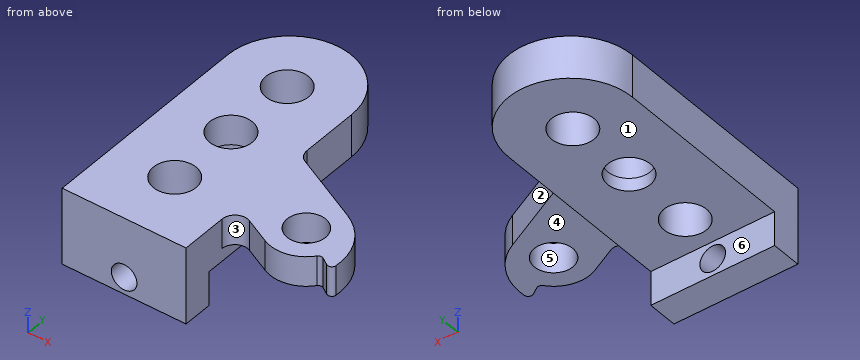
```python
from build123d import *

# Parameters (mm, degrees)
ESQUISSE1_R             = 5
ESQUISSE1_R_2           = 4.5
BOSS_EXTRU_1_DEPTH      = 7
ESQUISSE4_R             = 5
BOSS_EXTRU_3_DEPTH      = 3
ESQUISSE5_W             = 29
ESQUISSE5_H             = 7
BOSS_EXTRU_4_DEPTH      = 8
ESQUISSE6_R             = 3
ENL_V_MAT_EXTRU_1_DEPTH = 65.5
ESQUISSE8_R             = 5
ENL_V_MAT_EXTRU_2_DEPTH = 19


with BuildPart() as part:
    # Esquisse1 → Boss.-Extru.1 (new body)
    with BuildSketch(Plane.XY):
        with BuildLine():
            Line((-14.5, -25), (14.5, -25))
            Line((14.5, -25), (14.5, -14.109086144))
            ThreePointArc((14.5, -14.109086144), (15.91383086, -11.562702933), (18.822711639, -11.416423165))
            Line((18.822711639, -11.416423165), (24.752317023, -14.329211775))
            ThreePointArc((24.752317023, -14.329211775), (30.322333643, -15.002355093), (35.098387692, -12.05829076))
            ThreePointArc((35.098387692, -12.05829076), (35.719225888, -11.700832999), (36.419839787, -11.850353167))
            Line((36.419839787, -11.850353167), (38.096489271, -12.940695548))
            ThreePointArc((38.096489271, -12.940695548), (39.079315926, -13.001513562), (39.637771245, -12.190480443))
            ThreePointArc((39.637771245, -12.190480443), (37.976265411, -4.485178535), (32.247682977, 0.929211775))
            Line((32.247682977, 0.929211775), (16.177288361, 8.823440709))
            ThreePointArc((16.177288361, 8.823440709), (14.953616789, 9.929934548), (14.5, 11.516103688))
            Line((14.5, 11.516103688), (14.5, 25))
            ThreePointArc((14.5, 25), (0, 39.5), (-14.5, 25))
            Line((-14.5, 25), (-14.5, -25))
        make_face()
        with Locations((0, 7.3)):
            Circle(ESQUISSE1_R, mode=Mode.SUBTRACT)
        with Locations((28.5, -6.7)):
            Circle(ESQUISSE1_R_2, mode=Mode.SUBTRACT)
    extrude(amount=BOSS_EXTRU_1_DEPTH)

    # Esquisse4 → Boss.-Extru.3 (add)
    with BuildSketch(Plane(origin=(0, 0, 0), x_dir=(-1, 0, 0), z_dir=(0, 0, -1))):
        with BuildLine():
            Line((14.5, 25), (14.5, -25))
            Line((14.5, -25), (-14.5, -25))
            Line((-14.5, -25), (-14.5, 25))
            ThreePointArc((-14.5, 25), (0, 39.5), (14.5, 25))
        make_face()
        with Locations((0, 7.3)):
            Circle(ESQUISSE4_R, mode=Mode.SUBTRACT)
    extrude(amount=BOSS_EXTRU_3_DEPTH)

    # Esquisse5 → Boss.-Extru.4 (add)
    with BuildSketch(Plane(origin=(0, 0, -3), x_dir=(-1, 0, 0), z_dir=(0, 0, -1))):
        with Locations((0, -21.5)):
            Rectangle(ESQUISSE5_W, ESQUISSE5_H)
    extrude(amount=BOSS_EXTRU_4_DEPTH)

    # Esquisse6 → Enlèv. mat.-Extru.1 (cut, through all)
    with BuildSketch(Plane.XZ.offset(25)):
        with Locations(Location((0, -7, 0), (0, 0, 270))):  # turned: the seam where the file's is
            Circle(ESQUISSE6_R)
    extrude(amount=-ENL_V_MAT_EXTRU_1_DEPTH, mode=Mode.SUBTRACT)

    # Esquisse8 → Enlèv. mat.-Extru.2 (cut, through all)
    with BuildSketch(Plane.XY.offset(7)):
        with Locations((0, -9.7)):
            Circle(ESQUISSE8_R)
        with Locations((0, 24.3)):
            Circle(ESQUISSE8_R)
    extrude(amount=-ENL_V_MAT_EXTRU_2_DEPTH, mode=Mode.SUBTRACT)


solid = part.part
```
The model under review builds one solid part; all positions refer to its coordinate system, in mm. Face numbers are marked on the shaded views. A direction names the side the tool comes from. Give positions to 0.01 mm unless a question says otherwise; leave off trailing zeros. Write each loop counter-clockwise with the first axis right and the second up, starting at its lowest first coordinate (ties: lowest second). Pieces come first, ordered by that corner, then holes.
(1) The part is to be moulded in two halves that separate along X. For the marked faces 1, 2 and 3, say which applies: released by +X, released by -X, zero draft, split by the parting line, or undercut.
(2) For P1, Ø8, axis at x = 33, z = 4, coming from the -Y side; P2, Ø8.5, axis at x = -0.5, y = 5, coming from the -Z side; P3, Ø10.5, axis at x = 28.5, y = -6.7, coming from the -Z side, all flat-tipped, find the tip position at first contact; note any pin that passes through.
(3) Tool access review of the marked faces 4, 5 and 6: name each direction out of +Z, -Z, +X, -X, +Y, -Y from which nothing blocks a thin tool from reaching the whole face with its end or side.
(4) To check wall thickness, follow L1, parallel to Y at x = 0, z = 1.5; L2, parallel to X at y = 7.3, z = -0.85; L3, parallel to Z at x = 10.5, y = 7. State the ranges of each line that lie inside material, in increasing order.
(5) Consider section D-D, the plane x = 0. Give the boundary of the cut face in (y, z).
(6) Consider section B-B, the plane y = 24.3. Give the boundary of the cut face in (x, z), and give its area (3 significant figures).
(7) Consider section A-A, the plane z = -7. Give the boundary of the cut face in (x, y).
(8) Consider section C-C, the plane z = 1.75. Give the boundary of the cut face in (x, y).
Returned:
1. face 1: zero draft
1. face 2: released by +X
1. face 3: undercut
2. P1: stops at y = -15.19
2. P2: stops at z = -3
2. P3: stops at z = 0
3. face 4: -Z, +X, +Y, -Y
3. face 5: +Z, -Z
3. face 6: -Z, +X, -X, +Y
4. L1: y = -25 to -14.7, -4.7 to 2.3, 12.3 to 19.3, 29.3 to 39.5
4. L2: x = -14.5 to -5, 5 to 14.5
4. L3: z = -3 to 7
5. outline: (-25, -11) - (-18, -11) - (-18, -10) - (-25, -10) - close; (-25, -4) - (-18, -4) - (-18, -3) - (-14.7, -3) - (-14.7, 7) - (-25, 7) - close; (-4.7, -3) - (2.3, -3) - (2.3, 7) - (-4.7, 7) - close; (12.3, -3) - (19.3, -3) - (19.3, 7) - (12.3, 7) - close; (29.3, -3) - (39.5, -3) - (39.5, 7) - (29.3, 7) - close
6. outline: (-14.5, -3) - (-5, -3) - (-5, 7) - (-14.5, 7) - close; (5, -3) - (14.5, -3) - (14.5, 7) - (5, 7) - close
6. area: 190 mm2
7. outline: (-14.5, -25) - (-3, -25) - (-3, -18) - (-14.5, -18) - close; (3, -25) - (14.5, -25) - (14.5, -18) - (3, -18) - close
8. outline: (-14.5, -25) - (14.5, -25) - (14.5, -14.11) arc R3 cw to (18.82, -11.42) - (24.75, -14.33) arc R8.5 ccw to (35.1, -12.06) arc R1 cw to (36.42, -11.85) - (38.1, -12.94) arc R1 ccw to (39.64, -12.19) arc R13.31 ccw to (32.25, 0.93) - (16.18, 8.82) arc R3 cw to (14.5, 11.52) - (14.5, 25) arc R14.5 ccw to (-14.5, 25) - close; hole circle Ø10 at (0, -9.7); hole circle Ø10 at (0, 7.3); hole circle Ø10 at (0, 24.3); hole circle Ø9 at (28.5, -6.7)
